```python
from build123d import *

# Parameters (mm, degrees)
SZKIC1_W                    = 100
SZKIC1_H                    = 100
DODANIE_WYCI_GNI_CIE1_DEPTH = 4
DODANIE_WYCI_GNI_CIE5_DEPTH = 196


with BuildPart() as part:
    # Szkic1 → Dodanie-wyciągnięcie1 (new body)
    with BuildSketch(Plane.XY):
        with Locations((-50, 50)):
            Rectangle(SZKIC1_W, SZKIC1_H)
        with Locations((50, 50)):
            Rectangle(SZKIC1_W, SZKIC1_H)
        with Locations((50, -50)):
            Rectangle(SZKIC1_W, SZKIC1_H)
        with Locations((-50, -50)):
            Rectangle(SZKIC1_W, SZKIC1_H)
    extrude(amount=DODANIE_WYCI_GNI_CIE1_DEPTH)

    # Szkic2 → Dodanie-wyciągnięcie5 (add)
    with BuildSketch(Plane.XY.offset(4)):
        with BuildLine():
            Line((0, 100), (0, 75.322074641))
            ThreePointArc((0, 75.322074641), (27.168001538, 27.168001538), (75.322074641, 0))
            Line((75.322074641, 0), (100, 0))
            Line((100, 0), (100, 3))
            ThreePointArc((100, 3), (31.410642225, 31.410642225), (3, 100))
            Line((3, 100), (0, 100))
        make_face()
        with BuildLine():
            Line((100, 0), (75.322074641, 0))
            ThreePointArc((75.322074641, 0), (87.570197105, -2.247249352), (100, -3))
            Line((100, -3), (100, 0))
        make_face()
        with BuildLine():
            ThreePointArc((-3, 100), (-2.247249352, 87.570197105), (0, 75.322074641))
            Line((0, 75.322074641), (0, 100))
            Line((0, 100), (-3, 100))
        make_face()
    extrude(amount=DODANIE_WYCI_GNI_CIE5_DEPTH)


solid = part.part
```
Could you check a few things on this model? Use its own coordinates, in mm. A direction names the side the tool comes from. Round coordinates to 2 decimals unless told otherwise and drop trailing zeros. Loops run counter-clockwise (first coordinate to the right, second up) from the corner with the lowest first, then second, coordinate; pieces in that order, holes last. Notation, with made-up numbers: (-9, 64.5) - (10, 64.5) arc R22 ccw to (10, 70.5) - close; hole circle Ø1 at (-17, 40). An arc over 180 degrees is marked (long way). Use CSV: the item, a comma, the result in double quotes.
Item 1: If we section it at B-B on x = 34: List the corners of the cut face in (y, z) for me.
Here are the results:
outline,"(-100, 0) - (100, 0) - (100, 4) - (28.92, 4) - (28.92, 200) - (20.92, 200) - (20.92, 4) - (-100, 4) - close"
Item 2: If we section it at C-C on y = 17.5: List the corners of the cut face in (x, z) for me.
Here are the results:
outline,"(-100, 0) - (100, 0) - (100, 4) - (48.98, 4) - (48.98, 200) - (38.33, 200) - (38.33, 4) - (-100, 4) - close"
Item 3: I need wall thicknesses on L1, parallel to Z at x = 22.5, y = 15.5; L2, parallel to Y at x = 44, z = 23.5; L3, parallel to Y at x = 61, z = 44. Which ranges of each line are inside material? Lowest first, please. Write a range as [from, to].
Here are the results:
L1,"z = [0, 4]"
L2,"y = [13.55, 20.8]"
L3,"y = [4.67, 11.19]"
Item 4: If we mould it in two halves opening along Z, with no side actions, what happens to faces 1 (the flat face through (-24, -21, 4)), 2 (the flat face through (-1, 1, 0)), 3 (the flat face through (0, 100, 55))? For each: pulls with the +Z half, pulls with the -Z half, needs draft (parallel to the pull), parting line crosses it, or undercut.
Here are the results:
face 1,"pulls with the +Z half"
face 2,"pulls with the -Z half"
face 3,"needs draft"
Item 5: If we section it at D-D on y = -46.5: List the corners of the cut face in (x, z) for me.
Here are the results:
outline,"(-100, 0) - (100, 0) - (100, 4) - (-100, 4) - close"
Item 6: If we section it at A-A on z = 125.5: List the corners of the cut face in (x, y) for me, then the cut area to 3 significant figures.
Here are the results:
outline,"(-3, 100) arc R103 ccw to (100, -3) - (100, 3) arc R97 cw to (3, 100) - close"
area,"942 mm²"
Item 7: For faces 4 (the flat face through (29, 33, 200)), 5 (the flat face through (62, 63, 4)), which set-ups out of +Z, -Z, +X, -X, +Y, -Y let a thin tool reach every point of the face, with its end or its side?
Here are the results:
face 4,"+Z, +X, -X, +Y, -Y"
face 5,"+Z, +X, +Y"
Item 8: Will these pins go through, and if not, where does the flat tip stop? pin 1 (3 mm diameter, centred on y = -4, z = 67, fed in from +X); pin 2 (10 mm diameter, centred on x = -39.5, y = 47.5, fed in from +Z); pin 3 (2 mm diameter, centred on y = 76.5, z = 38, fed in from -X); pin 4 (10 mm diameter, centred on y = 69.5, z = 176, fed in from +X).
Here are the results:
pin 1,"stops at x = 100"
pin 2,"stops at z = 4"
pin 3,"stops at x = -0.51"
pin 4,"stops at x = 9.73"
